Geometry: final body of the model. Coordinates: model frame, mm. A direction names the side the tool comes from. Give positions to 0.01 mm unless a question says otherwise; leave off trailing zeros. Order: outer loops, then holes, each group sorted by start corner. A loop starts at its lowest first (then second) coordinate and runs counter-clockwise, first axis right, second up. Notation, with made-up numbers: (-1.5, 61) - (5.5, 61) arc R10 ccw to (5.5, 72) - close; hole circle Ø4 at (-34, 87.25). An arc over 180 degrees is marked (long way). Put each result on its own line as item: value. Start each with the question number.
1. Set-up query: faces 5 (the cylindrical face through (39.34, 0.89, 103.44)), 6 (the cylindrical face through (51.426, 24.227, 20.329)), 7 (the cylindrical face through (106.31, -8.27, 75.66)). Return all of +Z, -Z, +X, -X, +Y, -Y with unobstructed straight access to the full face (end or side cutting, diameter ignored); none if empty.
2. Ray query, line 1 along Z through (x, y) = (-3, 36); line 2 along X through (y, z) = (8.5, -41.5); line 3 along X through (y, z) = (54, 2). Return the intervals inside material, ascending. Write a range as from..to.
3. Mould query, pull axis X, two halves, no side actions, for faces 1 (the flat face through (-13, 1, 0)), 2 (the flat face through (50.8, -1, 44)), 3 (the flat face through (106.68, -1, 14)), 4 (the flat face through (0, -1, -56)). Classes: pulls with the +X half, pulls with the -X half, needs draft (parallel to the pull), parting line crosses it, or undercut.
4. First-contact query: P1, Ø1, axis at x = 27.5, y = 7.5, coming from the -Z side; P2, Ø4, axis at y = -37.5, z = -41.5, coming from the -X side; P3, Ø12, axis at x = 35.5, y = 46.5, coming from the -Z side. Flat tips, straight axial feed; report the tip coordinate or a pass-through.
5. Section A-A on z = -85. Return the cut outline in (x, y).
from build123d import *

# Parameters (mm, degrees)
F0_W      = 127
F0_H      = 228.6
F1_DEPTH  = 50.8
F2_R      = 38.1
F3_SIZE2  = 72.549909
F3_SIZE   = 50.79999
F4_W      = 127
F4_H      = 12.7
F5_DEPTH  = 25.4
F6_W      = 127
F6_H      = 101.6
F7_DEPTH  = 25.4
F8_R      = 25.4
F9_DEPTH  = 1.27
F10_R     = 63.5
F11_DEPTH = 54.61


# Not quite as in the source:
# - a fillet or chamfer that OpenCascade refuses, or shapes differently, is made with other operations: its cross-section is extruded or revolved along the edge and cut away or added
# - a fillet or chamfer is up to 0.001 mm smaller than in the source, because OpenCascade refuses the exact size


with BuildPart() as f1:
    # F0 (on Right) → F1 (new body)
    with BuildSketch(Plane.YZ):
        Rectangle(F0_W, F0_H)
    extrude(amount=F1_DEPTH)

    # F2
    f2_edges = [f1.edges().sort_by_distance(p)[0] for p in [
        (50.8, 0, 114.3),
    ]]
    fillet(f2_edges, radius=F2_R)

    # F3 (size 50.8 and 72.5499187425 in the source; OpenCascade refuses exactly that, so slightly less here)
    f3_edges = [f1.edges().sort_by_distance(p)[0] for p in [
        (50.8, 0, -114.3),
    ]]
    f3_side = f1.faces().sort_by_distance((25.4, 0, -114.3))[0]
    chamfer(f3_edges, length=F3_SIZE, length2=F3_SIZE2, reference=f3_side)

    # F4 (on face) → F5 (join)
    with BuildSketch(Plane(origin=(0, 0, 0), x_dir=(0, -1, 0), z_dir=(-1, 0, 0))):
        with Locations((0, 107.95)):
            Rectangle(F4_W, F4_H)
    extrude(amount=F5_DEPTH)

    # F6 (on face) → F7 (join)
    with BuildSketch(Plane(origin=(0, 0, 0), x_dir=(0, -1, 0), z_dir=(-1, 0, 0))):
        with Locations((0, 50.8)):
            Rectangle(F6_W, F6_H)
    extrude(amount=F7_DEPTH)

    # F8 (on face) → F9 (join)
    with BuildSketch(Plane.YZ.offset(50.8)):
        with Locations((0, 12.7)):
            Circle(F8_R)
    extrude(amount=F9_DEPTH)

    # F10 (on face) → F11 (join)
    with BuildSketch(Plane.YZ.offset(52.07)):
        with Locations((0, 12.7)):
            Circle(F10_R)
    extrude(amount=F11_DEPTH)

    # F12: fillet of radius 57.15 on 1 edges, made by hand

    # F12_s1 → F12_t2 (revolve, cut)
    with BuildSketch(Plane.XY.offset(12.7)):
        with BuildLine():
            ThreePointArc((105.9515367264, 63.5), (72.9559688422, 53.0127796), (52.07, 25.4))
            Line((52.07, 25.4), (52.07, 63.5))
            Line((52.07, 63.5), (105.9515367264, 63.5))
        make_face()
    revolve(axis=Axis((52.07, 0, 12.7), (1, 0, 0)), mode=Mode.SUBTRACT)


solid = f1.part
Resolved:
1. face 5: +Z, +X, +Y, -Y
1. face 6: none
1. face 7: +X
2. line 1: 0..114.3
2. line 2: 0..50.8, 75.74..106.68
2. line 3: -25.4..50.8, 76.04..106.68
3. face 1: needs draft
3. face 2: undercut
3. face 3: pulls with the +X half
3. face 4: pulls with the -X half
4. P1: z = -75.74
4. P2: x = 0
4. P3: z = -72.17
5. outline: (0, -63.5) - (20.52, -63.5) - (20.52, 63.5) - (0, 63.5) - close
